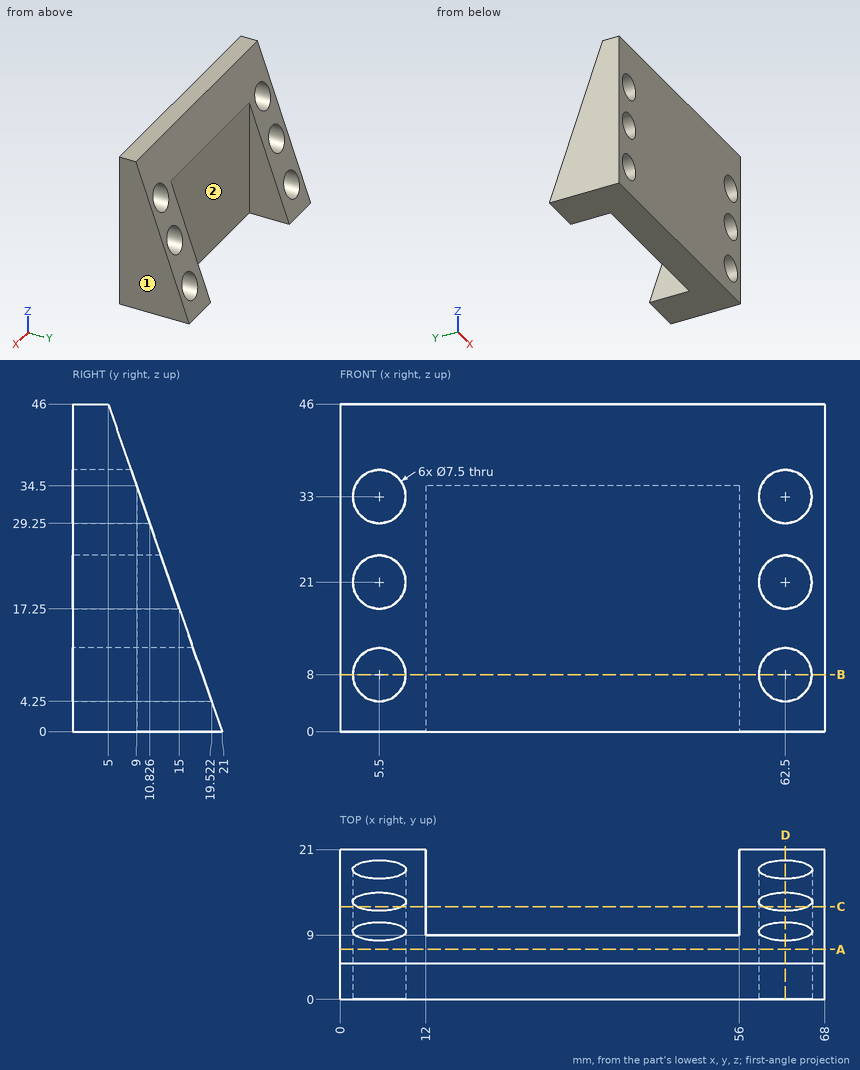
Input: dimensioned drawing with shaded views. Units: mm. Origin: part minimum x, y, z. A direction names the side the tool comes from. Round coordinates to 2 decimals unless told otherwise and drop trailing zeros. Loops run counter-clockwise (first coordinate to the right, second up) from the corner with the lowest first, then second, coordinate; pieces in that order, holes last. Notation, with made-up numbers: (-35, 52) -> (-8, 52) arc R26 cw to (-8, 80) -> close; hole circle Ø1 at (29, 33). An arc over 180 degrees is marked (long way). Answer as a JSON object with one key per item and string values. Group by question number.
Q1. Section query B-B (z = 8). Output: boundary loops of the cut face in (x, y), plus the area to 3 significant figures.
Q2. Section query A-A (y = 7). Output: boundary loops of the cut face in (x, z).
Q3. Section query C-C (y = 13). Output: boundary loops of the cut face in (x, z), plus the area to 3 significant figures.
Q4. Section query D-D (x = 62.5). Output: boundary loops of the cut face in (y, z), plus the area to 3 significant figures.
Q5. Access query for the marked faces 1 and 2. Directions: +Z, -Z, +X, -X, +Y, -Y. A direction counts if a zero-diameter tool reaches every point of the face in a straight line with its end or side. Return the directions, or none.
Q6. Contact query for flat-ended pins moving along their axis: P1, Ø4.5, axis at x = 5.5, z = 8, coming from the +Y side; P2, Ø3, axis at x = 17.5, z = 22.5, coming from the +Y side; P3, Ø2, axis at x = 37, z = 39.5, coming from the +Y side. Output: stop coordinate, or through.
Q7. Ray query, line 1 (X direction, y = 7.75, z = 21); line 2 (X direction, y = 9.5, z = 21); line 3 (X direction, y = 8.75, z = 6). Return the intervals inside material, ascending. Write a range as from..to.
Completed:
{
 "1": {"outline": "(0, 0) -> (1.75, 0) -> (1.75, 18.22) -> (0, 18.22) -> close; (9.25, 0) -> (58.75, 0) -> (58.75, 18.22) -> (56, 18.22) -> (56, 9) -> (12, 9) -> (12, 18.22) -> (9.25, 18.22) -> close; (66.25, 0) -> (68, 0) -> (68, 18.22) -> (66.25, 18.22) -> close", "area": "560 mm²"},
 "2": {"outline": "(0, 0) -> (68, 0) -> (68, 40.25) -> (0, 40.25) -> close; hole circle Ø7.5 at (5.5, 8); hole circle Ø7.5 at (5.5, 21); hole circle Ø7.5 at (5.5, 33); hole circle Ø7.5 at (62.5, 8); hole circle Ø7.5 at (62.5, 21); hole circle Ø7.5 at (62.5, 33)"},
 "3": {"outline": "(0, 0) -> (12, 0) -> (12, 23) -> (8.67, 23) arc R3.75 cw (long way) to (2.33, 23) -> (0, 23) -> close; (56, 0) -> (68, 0) -> (68, 23) -> (65.67, 23) arc R3.75 cw (long way) to (59.33, 23) -> (56, 23) -> close; hole circle Ø7.5 at (5.5, 8); hole circle Ø7.5 at (62.5, 8)", "area": "391 mm²"},
 "4": {"outline": "(0, 0) -> (21, 0) -> (19.52, 4.25) -> (0, 4.25) -> close; (0, 11.75) -> (16.91, 11.75) -> (15, 17.25) -> (0, 17.25) -> close; (0, 24.75) -> (12.39, 24.75) -> (10.83, 29.25) -> (0, 29.25) -> close; (0, 36.75) -> (8.22, 36.75) -> (5, 46) -> (0, 46) -> close", "area": "287 mm²"},
 "5": {"face 1": "+Z, -Z, +X, +Y, -Y", "face 2": "+Z, -Z, +Y"},
 "6": {"P1": "through", "P2": "y = 9", "P3": "y = 7.61"},
 "7": {"line 1": "0..1.75, 9.25..58.75, 66.25..68", "line 2": "0..1.75, 9.25..12, 56..58.75, 66.25..68", "line 3": "0..2.33, 8.67..59.33, 65.67..68"}
}
